from build123d import *

# Parameters (mm, degrees)
BOSS_EXTRUDE1_REACH      = 43.243
BOSS_EXTRUDE1_END_RADIUS = 18
SKETCH4_W                = 4.5
SKETCH4_H                = 2
FILLET1_R                = 4


with BuildPart() as part:
    # Sweep1: sweep along a path in Sketch1
    with BuildLine(Plane(origin=(0, 0, 0), x_dir=(1, 0, 0), z_dir=(0, 1, 0))) as sweep1_path:
        Line((-4.5, 18), (-4.5, 11.9058809))
        ThreePointArc((-4.5, 11.9058809), (-5.08127088, 8.723900384), (-6.75, 5.95294045))
        ThreePointArc((-6.75, 5.95294045), (0, -9), (6.75, 5.95294045))
        ThreePointArc((6.75, 5.95294045), (5.08127088, 8.723900384), (4.5, 11.9058809))
        Line((4.5, 11.9058809), (4.5, 18))
    # Sketch3 → Sweep1 (sweep)
    with BuildSketch(Plane(origin=(0, 0, 0), x_dir=(0, 0, -1), z_dir=(1, 0, 0))):
        with BuildLine():
            Line((-18, 9), (-15, 9))
            ThreePointArc((-15, 9), (-10.757359313, 7.242640687), (-9, 3))
            Line((-9, 3), (-9, 0))
            Line((-9, 0), (-9, -3))
            ThreePointArc((-9, -3), (-10.757359313, -7.242640687), (-15, -9))
            Line((-15, -9), (-18, -9))
            Line((-18, -9), (-18, -7))
            Line((-18, -7), (-15, -7))
            ThreePointArc((-15, -7), (-12.171572875, -5.828427125), (-11, -3))
            Line((-11, -3), (-11, 3))
            ThreePointArc((-11, 3), (-12.171572875, 5.828427125), (-15, 7))
            Line((-15, 7), (-18, 7))
            Line((-18, 7), (-18, 9))
        make_face()
    sweep(path=sweep1_path.line)

    # Boss-Extrude1: up to this cylinder (the profile starts outside it)
    boss_extrude1_end = Plane(origin=(0, 0, 0), z_dir=(0, 1, 0)) * Cylinder(BOSS_EXTRUDE1_END_RADIUS, 139.486, mode=Mode.PRIVATE)
    # Sketch4 → Boss-Extrude1 (add, up to the surface)
    with BuildSketch(Plane(origin=(0, 0, -18), x_dir=(-1, 0, 0), z_dir=(0, 0, -1)), mode=Mode.PRIVATE) as boss_extrude1_sk1:
        with Locations((-15.75, 8)):
            Rectangle(SKETCH4_W, SKETCH4_H)
    boss_extrude1_tool1 = extrude(boss_extrude1_sk1.sketch, amount=-BOSS_EXTRUDE1_REACH, mode=Mode.PRIVATE) - boss_extrude1_end
    add(boss_extrude1_tool1.solids().sort_by_distance((15.75, 8, -18))[0])
    # Sketch4 → Boss-Extrude1 (add, up to the surface)
    with BuildSketch(Plane(origin=(0, 0, -18), x_dir=(-1, 0, 0), z_dir=(0, 0, -1)), mode=Mode.PRIVATE) as boss_extrude1_sk2:
        with Locations((15.75, 8)):
            Rectangle(SKETCH4_W, SKETCH4_H)
    boss_extrude1_tool2 = extrude(boss_extrude1_sk2.sketch, amount=-BOSS_EXTRUDE1_REACH, mode=Mode.PRIVATE) - boss_extrude1_end
    add(boss_extrude1_tool2.solids().sort_by_distance((-15.75, 8, -18))[0])
    # Sketch4 → Boss-Extrude1 (add, up to the surface)
    with BuildSketch(Plane(origin=(0, 0, -18), x_dir=(-1, 0, 0), z_dir=(0, 0, -1)), mode=Mode.PRIVATE) as boss_extrude1_sk3:
        with Locations((15.75, -8)):
            Rectangle(SKETCH4_W, SKETCH4_H)
    boss_extrude1_tool3 = extrude(boss_extrude1_sk3.sketch, amount=-BOSS_EXTRUDE1_REACH, mode=Mode.PRIVATE) - boss_extrude1_end
    add(boss_extrude1_tool3.solids().sort_by_distance((-15.75, -8, -18))[0])
    # Sketch4 → Boss-Extrude1 (add, up to the surface)
    with BuildSketch(Plane(origin=(0, 0, -18), x_dir=(-1, 0, 0), z_dir=(0, 0, -1)), mode=Mode.PRIVATE) as boss_extrude1_sk4:
        with Locations((-15.75, -8)):
            Rectangle(SKETCH4_W, SKETCH4_H)
    boss_extrude1_tool4 = extrude(boss_extrude1_sk4.sketch, amount=-BOSS_EXTRUDE1_REACH, mode=Mode.PRIVATE) - boss_extrude1_end
    add(boss_extrude1_tool4.solids().sort_by_distance((15.75, -8, -18))[0])

    # Fillet1
    fillet1_edges = [part.edges().sort_by_distance(p)[0] for p in [
        (18, -8, -18),
        (-18, -8, -18),
        (-18, 8, -18),
        (18, 8, -18),
    ]]
    fillet(fillet1_edges, radius=FILLET1_R)


solid = part.part
Input: part model. Units: mm. Frame: model coordinates. A direction names the side the tool comes from. Round coordinates to 2 decimals unless told otherwise and drop trailing zeros. Write each loop counter-clockwise with the first axis right and the second up, starting at its lowest first coordinate (ties: lowest second). Pieces come first, ordered by that corner, then holes.
1) Cut plane C-C (y = -0.25). Return the cut outline in (x, z).
2) Ray query, L1, parallel to X at y = -1.35, z = 0; L2, parallel to X at y = 1.75, z = -16; L3, parallel to Y at x = -8.5, z = 14. Return the intervals inside material, ascending.
3) Draft query along X for faces 6 (the cylindrical face through (0, 8, 18)), 7 (the cylindrical face through (-6.211, 7.196, -14.91)), 8 (the cylindrical face through (-16.797, 8.014, -16.859)). Return one class per face: pulls with the +X half, pulls with the -X half, needs draft (parallel to the pull), parting line crosses it, or undercut.
4) Cut plane B-B (x = 0). Return the cut outline in (y, z).
5) Cut plane A-A (z = -14.5). Return the cut outline in (x, y).
6) Contact query for flat-ended pins moving along their axis: P1, Ø3, axis at y = 0, z = -16, coming from the -X side; P2, Ø1.8, axis at y = -0.5, z = -14.5, coming from the +X side; P3, Ø1, axis at y = 4, z = 6.5, coming from the -X side. Output: stop coordinate, or through.
7) Reachability of faces 1 (the cylindrical face through (-6.94, -0.04, -9.46)), 2 (the flat face through (4.5, 0, -15)), 3 (the cylindrical face through (-6.304, -7.289, -14.91)), 4 (the flat face through (6.5, 0, -15)), 5 (the flat face through (13, -7, -8)) from +Z, -Z, +X, -X, +Y, -Y: full face, straight path, thin tool, end or side. Return the list, or none.
Geometry says:
1. outline: (-8.25, -7.28) arc R7 cw to (-6.5, -11.91) - (-6.5, -18) - (-4.5, -18) - (-4.5, -11.91) arc R9 ccw to (-6.75, -5.95) arc R9 cw (long way) to (6.75, -5.95) arc R9 ccw to (4.5, -11.91) - (4.5, -18) - (6.5, -18) - (6.5, -11.91) arc R7 cw to (8.25, -7.28) arc R11 ccw (long way) to start
2. L1: x = -11 to -9, 9 to 11
2. L2: x = -6.5 to -4.5, 4.5 to 6.5
2. L3: y = -9 to -7, 7 to 9
3. face 6: parting line crosses it
3. face 7: undercut
3. face 8: pulls with the -X half
4. outline: (-9, 15) arc R6 ccw to (-3, 9) - (3, 9) arc R6 ccw to (9, 15) - (9, 18) - (7, 18) - (7, 15) arc R4 cw to (3, 11) - (-3, 11) arc R4 cw to (-7, 15) - (-7, 18) - (-9, 18) - close
5. outline: (-17.97, -9) - (-10.5, -9) arc R6 ccw to (-4.5, -3) - (-4.5, 3) arc R6 ccw to (-10.5, 9) - (-17.97, 9) - (-17.97, 7) - (-10.5, 7) arc R4 cw to (-6.5, 3) - (-6.5, -3) arc R4 cw to (-10.5, -7) - (-17.97, -7) - close; (4.5, -3) arc R6 ccw to (10.5, -9) - (17.97, -9) - (17.97, -7) - (10.5, -7) arc R4 cw to (6.5, -3) - (6.5, 3) arc R4 cw to (10.5, 7) - (17.97, 7) - (17.97, 9) - (10.5, 9) arc R6 ccw to (4.5, 3) - close
6. P1: stops at x = -6.5
6. P2: stops at x = 6.5
6. P3: stops at x = -9.41
7. face 1: -Z, -X
7. face 2: -Z, +Y, -Y
7. face 3: -Z, -Y
7. face 4: -Z, +X
7. face 5: none
